CAD build for the part. Positions are in the model's coordinates, mm. Face numbers are marked on the shaded views. A direction names the side the tool comes from. Give positions to 0.01 mm unless a question says otherwise; leave off trailing zeros. Write each loop counter-clockwise with the first axis right and the second up, starting at its lowest first coordinate (ties: lowest second). Pieces come first, ordered by that corner, then holes. Notation, with made-up numbers: (-16, 60) - (9, 60) arc R29 cw to (9, 83) - close; hole circle Ø1 at (-9, 59). An arc over 180 degrees is marked (long way). Put each result on its own line as item: value. Start each with the question number.
1. Tool access for the marked faces 1, 2 and 3: list every direction of +Z, -Z, +X, -X, +Y, -Y with a clear straight run to the whole face (end or side of a thin tool).
2. Cut at D-D on x = -12. List the corners of the cut face in (y, z), and give its area (3 significant figures).
3. Cut at C-C on z = 12.75. List the corners of the cut face in (x, y).
4. Drop flat-ended pins along their axis: pin 1 (5 mm diameter, centred on x = -18, z = 7, fed in from -Y); pin 2 (5 mm diameter, centred on x = -15, z = 9, fed in from +Y); pin 3 (4 mm diameter, centred on y = 15, z = 7, fed in from +X). Give the stop position or say it passes through.
5. Mould opens along Y. For the marked faces 4, 5, 6 and 7 say: +Y half, -Y half, draft (parallel to the pull), parting line (faces both ways), or undercut.
6. Wall check: line 1 (Y direction, x = 0, z = 11.25); line 2 (Y direction, x = 7.5, z = 1.75); line 3 (X direction, y = -11.5, z = 2.5). Give the ranges that are in metal, low to high.
7. Cut at A-A on y = 0. List the corners of the cut face in (x, z), and give its area (3 significant figures).
from build123d import *

# Parameters (mm, degrees)
SKETCH1_R      = 23.5
EXTRUDE1_DEPTH = 14
SKETCH2_R      = 19.5
SKETCH2_R_2    = 14.25
EXTRUDE2_DEPTH = 5
SKETCH3_R      = 19.5
SKETCH3_R_2    = 14.25
EXTRUDE3_DEPTH = 5
SKETCH4_R      = 10
EXTRUDE4_DEPTH = 15


with BuildPart() as part:
    # Sketch1 → Extrude1 (new body)
    with BuildSketch(Plane.XY):
        Circle(SKETCH1_R)
    extrude(amount=EXTRUDE1_DEPTH)

    # Sketch2 → Extrude2 (cut)
    with BuildSketch(Plane.XY.offset(14)):
        Circle(SKETCH2_R)
        Circle(SKETCH2_R_2, mode=Mode.SUBTRACT)
    extrude(amount=-EXTRUDE2_DEPTH, mode=Mode.SUBTRACT)

    # Sketch3 → Extrude3 (cut)
    with BuildSketch(Plane(origin=(0, 0, 0), x_dir=(-1, 0, 0), z_dir=(0, 0, -1))):
        Circle(SKETCH3_R)
        Circle(SKETCH3_R_2, mode=Mode.SUBTRACT)
    extrude(amount=-EXTRUDE3_DEPTH, mode=Mode.SUBTRACT)

    # Sketch4 → Extrude4 (cut, through all)
    with BuildSketch(Plane(origin=(0, 0, 0), x_dir=(-1, 0, 0), z_dir=(0, 0, -1))):
        Circle(SKETCH4_R)
    extrude(amount=-EXTRUDE4_DEPTH, mode=Mode.SUBTRACT)


solid = part.part
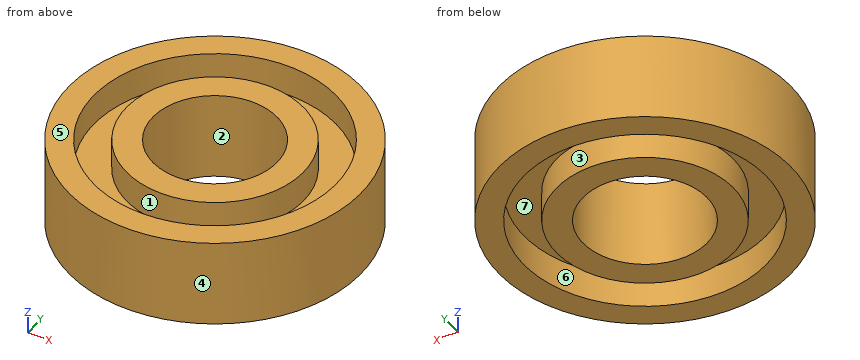
Report:
1. face 1: +Z
1. face 2: +Z, -Z
1. face 3: -Z
2. outline: (-20.21, 0) - (-15.37, 0) - (-15.37, 5) - (-7.69, 5) - (-7.69, 0) - (7.69, 0) - (7.69, 5) - (15.37, 5) - (15.37, 0) - (20.21, 0) - (20.21, 14) - (15.37, 14) - (15.37, 9) - (7.69, 9) - (7.69, 14) - (-7.69, 14) - (-7.69, 9) - (-15.37, 9) - (-15.37, 14) - (-20.21, 14) - close
2. area: 412 mm²
3. outline: circle Ø47 at (0, 0); circle Ø28.5 at (0, 0); hole circle Ø39 at (0, 0); hole circle Ø20 at (0, 0)
4. pin 1: stops at y = -17.66
4. pin 2: stops at y = 19.9
4. pin 3: stops at x = 19.58
5. face 4: parting line
5. face 5: draft
5. face 6: undercut
5. face 7: undercut
6. line 1: y = -23.5 to -19.5, -14.25 to -10, 10 to 14.25, 19.5 to 23.5
6. line 2: y = -22.27 to -18, -12.12 to -6.61, 6.61 to 12.12, 18 to 22.27
6. line 3: x = -20.49 to -15.75, -8.42 to 8.42, 15.75 to 20.49
7. outline: (-23.5, 0) - (-19.5, 0) - (-19.5, 5) - (-14.25, 5) - (-14.25, 0) - (-10, 0) - (-10, 14) - (-14.25, 14) - (-14.25, 9) - (-19.5, 9) - (-19.5, 14) - (-23.5, 14) - close; (10, 0) - (14.25, 0) - (14.25, 5) - (19.5, 5) - (19.5, 0) - (23.5, 0) - (23.5, 14) - (19.5, 14) - (19.5, 9) - (14.25, 9) - (14.25, 14) - (10, 14) - close
7. area: 273 mm²
